from build123d import *

# Parameters (mm, degrees)
ESQUISSE1_W                     = 350
ESQUISSE1_H                     = 360
ESQUISSE1_W_2                   = 60
ESQUISSE1_H_2                   = 60
BOSS_EXTRU_1_DEPTH              = 3
ESQUISSE2_R                     = 3.175
ENL_V_MAT_EXTRU_1_DEPTH         = 5
ESQUISSE2_2_R                   = 4.175
ESQUISSE2_2_R_2                 = 3.175
ENL_V_DE_MAT_EXTRU_MINCE1_DEPTH = 1


with BuildPart() as part:
    # Esquisse1 → Boss.-Extru.1 (new body)
    with BuildSketch(Plane(origin=(0, 0, 0), x_dir=(1, 0, 0), z_dir=(0, 1, 0))):
        with Locations((155, 160)):
            Rectangle(ESQUISSE1_W, ESQUISSE1_H)
        with Locations((50, 50)):
            Rectangle(ESQUISSE1_W_2, ESQUISSE1_H_2, mode=Mode.SUBTRACT)
        with Locations((50, 120)):
            Rectangle(ESQUISSE1_W_2, ESQUISSE1_H_2, mode=Mode.SUBTRACT)
        with Locations((120, 120)):
            Rectangle(ESQUISSE1_W_2, ESQUISSE1_H_2, mode=Mode.SUBTRACT)
        with Locations((120, 50)):
            Rectangle(ESQUISSE1_W_2, ESQUISSE1_H_2, mode=Mode.SUBTRACT)
        with Locations((190, 50)):
            Rectangle(ESQUISSE1_W_2, ESQUISSE1_H_2, mode=Mode.SUBTRACT)
        with Locations((190, 120)):
            Rectangle(ESQUISSE1_W_2, ESQUISSE1_H_2, mode=Mode.SUBTRACT)
        with Locations((260, 120)):
            Rectangle(ESQUISSE1_W_2, ESQUISSE1_H_2, mode=Mode.SUBTRACT)
        with Locations((260, 50)):
            Rectangle(ESQUISSE1_W_2, ESQUISSE1_H_2, mode=Mode.SUBTRACT)
        with Locations((260, 260)):
            Rectangle(ESQUISSE1_W_2, ESQUISSE1_H_2, mode=Mode.SUBTRACT)
        with Locations((260, 190)):
            Rectangle(ESQUISSE1_W_2, ESQUISSE1_H_2, mode=Mode.SUBTRACT)
        with Locations((190, 190)):
            Rectangle(ESQUISSE1_W_2, ESQUISSE1_H_2, mode=Mode.SUBTRACT)
        with Locations((190, 260)):
            Rectangle(ESQUISSE1_W_2, ESQUISSE1_H_2, mode=Mode.SUBTRACT)
        with Locations((120, 260)):
            Rectangle(ESQUISSE1_W_2, ESQUISSE1_H_2, mode=Mode.SUBTRACT)
        with Locations((120, 190)):
            Rectangle(ESQUISSE1_W_2, ESQUISSE1_H_2, mode=Mode.SUBTRACT)
        with Locations((50, 190)):
            Rectangle(ESQUISSE1_W_2, ESQUISSE1_H_2, mode=Mode.SUBTRACT)
        with Locations((50, 260)):
            Rectangle(ESQUISSE1_W_2, ESQUISSE1_H_2, mode=Mode.SUBTRACT)
    extrude(amount=BOSS_EXTRU_1_DEPTH)

    # Esquisse2 → Enl_v. mat.-Extru.1 (cut)
    with BuildSketch(Plane(origin=(0, 3, 0), x_dir=(1, 0, 0), z_dir=(0, 1, 0))):
        with Locations((155, 300)):
            Circle(ESQUISSE2_R)
        with Locations((10, 300)):
            Circle(ESQUISSE2_R)
        with Locations((155, 155)):
            Circle(ESQUISSE2_R)
        with Locations((300, 300)):
            Circle(ESQUISSE2_R)
        with Locations((300, 155)):
            Circle(ESQUISSE2_R)
        with Locations((10, 155)):
            Circle(ESQUISSE2_R)
        with Locations((10, 10)):
            Circle(ESQUISSE2_R)
        with Locations((300, 10)):
            Circle(ESQUISSE2_R)
        with Locations((155, 10)):
            Circle(ESQUISSE2_R)
    extrude(amount=-ENL_V_MAT_EXTRU_1_DEPTH, mode=Mode.SUBTRACT)

    # Esquisse2_2 → Enl_v. de mat.-Extru.-Mince1 (cut)
    with BuildSketch(Plane(origin=(0, 3, 0), x_dir=(1, 0, 0), z_dir=(0, 1, 0))):
        with Locations((155, 300)):
            Circle(ESQUISSE2_2_R)
        with Locations((155, 300)):
            Circle(ESQUISSE2_2_R_2, mode=Mode.SUBTRACT)
        with Locations((10, 300)):
            Circle(ESQUISSE2_2_R)
        with Locations((10, 300)):
            Circle(ESQUISSE2_2_R_2, mode=Mode.SUBTRACT)
        with Locations((155, 155)):
            Circle(ESQUISSE2_2_R)
        with Locations((155, 155)):
            Circle(ESQUISSE2_2_R_2, mode=Mode.SUBTRACT)
        with Locations((300, 300)):
            Circle(ESQUISSE2_2_R)
        with Locations((300, 300)):
            Circle(ESQUISSE2_2_R_2, mode=Mode.SUBTRACT)
        with Locations((300, 155)):
            Circle(ESQUISSE2_2_R)
        with Locations((300, 155)):
            Circle(ESQUISSE2_2_R_2, mode=Mode.SUBTRACT)
        with Locations((10, 155)):
            Circle(ESQUISSE2_2_R)
        with Locations((10, 155)):
            Circle(ESQUISSE2_2_R_2, mode=Mode.SUBTRACT)
        with Locations((10, 10)):
            Circle(ESQUISSE2_2_R)
        with Locations((10, 10)):
            Circle(ESQUISSE2_2_R_2, mode=Mode.SUBTRACT)
        with Locations((300, 10)):
            Circle(ESQUISSE2_2_R)
        with Locations((300, 10)):
            Circle(ESQUISSE2_2_R_2, mode=Mode.SUBTRACT)
        with Locations((155, 10)):
            Circle(ESQUISSE2_2_R)
        with Locations((155, 10)):
            Circle(ESQUISSE2_2_R_2, mode=Mode.SUBTRACT)
    extrude(amount=-ENL_V_DE_MAT_EXTRU_MINCE1_DEPTH, mode=Mode.SUBTRACT)


solid = part.part
Source: CAD feature listing. Evaluate the final solid. Frame: model axes, mm. Give positions to 0.01 mm unless a question says otherwise; leave off trailing zeros. Order: outer loops, then holes, each group sorted by start corner. A loop starts at its lowest first (then second) coordinate and runs counter-clockwise, first axis right, second up. Notation, with made-up numbers: (-10.75, 5.25) -> (41.25, 5.25) arc R29 cw to (41.25, 39.25) -> close; hole circle Ø2 at (21.5, 86). An arc over 180 degrees is marked (long way). Write item = value, one per line.
Q1. Cut plane C-C, the plane y = 1.3. State how many separate pieces and enclosed holes the cut face has, and give its area (3 significant figures).
Data:
separate_pieces = 1
enclosed_holes = 25
area = 68,100 mm^2
Q2. Material intervals for line 1 (Z direction, x = 50.5, y = 0.9); line 2 (X direction, y = 2.3, z = -65); line 3 (Z direction, x = 300, y = 2.85) (3 decimals), sorted ascending. Write a range as from..to.
Data:
line_1 = -340..-290, -230..-220, -160..-150, -90..-80, -20..20
line_2 = -20..20, 80..90, 150..160, 220..230, 290..330
line_3 = -340..-304.175, -295.825..-159.175, -150.825..-14.175, -5.825..20
Q3. Cut plane B-B, the plane x = 241. Output: boundary loops of the cut face in (y, z).
Data:
outline = (0, -340) -> (3, -340) -> (3, -290) -> (0, -290) -> close; (0, -230) -> (3, -230) -> (3, -220) -> (0, -220) -> close; (0, -160) -> (3, -160) -> (3, -150) -> (0, -150) -> close; (0, -90) -> (3, -90) -> (3, -80) -> (0, -80) -> close; (0, -20) -> (3, -20) -> (3, 20) -> (0, 20) -> close
Q4. Pull-direction query (X, two-part tool) for faces 1 (the face through (303, 2, -157)), 2 (the face through (153, 3, -163)); classes: released by +X, released by -X, zero draft, split by the parting line, or undercut.
Data:
face_1 = undercut
face_2 = zero draft
Q5. Cut plane A-A, the plane z = -100. Output: boundary loops of the cut face in (x, y), and give its area (3 significant figures).
Data:
outline = (-20, 0) -> (20, 0) -> (20, 3) -> (-20, 3) -> close; (80, 0) -> (90, 0) -> (90, 3) -> (80, 3) -> close; (150, 0) -> (160, 0) -> (160, 3) -> (150, 3) -> close; (220, 0) -> (230, 0) -> (230, 3) -> (220, 3) -> close; (290, 0) -> (330, 0) -> (330, 3) -> (290, 3) -> close
area = 330 mm^2
Q6. Pin query (flat end, axial travel): pin 1 (1.5 mm diameter, centred on x = 227.5, z = -82.5, fed in from -Y); pin 2 (4 mm diameter, centred on x = 12, z = -300.5, fed in from +Y). Return the tip coordinate at first contact, or that it passes through.
Data:
pin_1 = 0
pin_2 = 2
